Geometry check sheet. Reference: the model listing, model coordinates, mm. Give positions to 0.01 mm unless a question says otherwise; leave off trailing zeros. Write each loop counter-clockwise with the first axis right and the second up, starting at its lowest first coordinate (ties: lowest second). Pieces come first, ordered by that corner, then holes.
(1) Cross-section at D-D (y = -51). Record the boundary of the cut face in (x, z), and give its area (3 significant figures).
(2) Cross-section at A-A (x = 48). Record the boundary of the cut face in (y, z), and give its area (3 significant figures).
(3) Thickness scan on line 1 along Y through (x, z) = (48, 0.3); line 2 along Y through (x, z) = (19, 0.65); line 3 along X through (y, z) = (-25.5, 0.65). Record the ranges inside material, lowest first.
(4) Depth check by flat-ended pin: P1, Ø1.7, axis at x = 48, y = -32.46, coming from the +Z side; P2, Ø0.5, axis at y = -39, z = 0.5, coming from the -X side. Enter the tip coordinate at first touch or a pass-through.
(5) Mould release check, pull along X, two halves, no side actions. Record for faces 1 (the cylindrical face through (18.902, -29.176, 0.507)), 2 (the flat face through (34, -21, 1)): +X half, -X half, draft (parallel to the pull), parting line (faces both ways), or undercut.
(6) Cross-section at B-B (z = 0.85). Count the separate pieces of the cut face and the enclosed holes in it, and give its area (3 significant figures).
(7) Cross-section at C-C (y = -29.92). Record the boundary of the cut face in (x, z), and give its area (3 significant figures).
```python
from build123d import *

# Parameters (mm, degrees)
IZIM1_R                     = 1.6
Y_KSEKLIK_EKSTR_ZYON1_DEPTH = 1
IZIM2_R                     = 0.75
KES_EKSTR_ZYON1_DEPTH       = 10


with BuildPart() as part:
    # Çizim1 → Yükseklik-Ekstrüzyon1 (new body)
    with BuildSketch(Plane.XY):
        Polygon((0, 0), (68, 0), (68, -17), (51, -17), (51, -54), (17, -54), (17, -17), (0, -17), align=None)
        with Locations((3, -8)):
            Circle(IZIM1_R, mode=Mode.SUBTRACT)
        with Locations((66, -8)):
            Circle(IZIM1_R, mode=Mode.SUBTRACT)
        with Locations((20, -51)):
            Circle(IZIM1_R, mode=Mode.SUBTRACT)
        with Locations((48, -51)):
            Circle(IZIM1_R, mode=Mode.SUBTRACT)
    extrude(amount=Y_KSEKLIK_EKSTR_ZYON1_DEPTH)

    # Çizim2 → Kes-Ekstrüzyon1 (cut)
    with BuildSketch(Plane.XY.offset(1)):
        with Locations((19, -35)):
            Circle(IZIM2_R)
        with Locations((19, -32.46)):
            Circle(IZIM2_R)
        with Locations((19, -29.92)):
            Circle(IZIM2_R)
        with Locations((48, -29.92)):
            Circle(IZIM2_R)
        with Locations((48, -32.46)):
            Circle(IZIM2_R)
        with Locations((48, -35)):
            Circle(IZIM2_R)
    extrude(amount=-KES_EKSTR_ZYON1_DEPTH, mode=Mode.SUBTRACT)


solid = part.part
```
Reply:
1. outline: (17, 0) - (18.4, 0) - (18.4, 1) - (17, 1) - close; (21.6, 0) - (46.4, 0) - (46.4, 1) - (21.6, 1) - close; (49.6, 0) - (51, 0) - (51, 1) - (49.6, 1) - close
1. area: 27.6 mm2
2. outline: (-54, 0) - (-52.6, 0) - (-52.6, 1) - (-54, 1) - close; (-49.4, 0) - (-35.75, 0) - (-35.75, 1) - (-49.4, 1) - close; (-34.25, 0) - (-33.21, 0) - (-33.21, 1) - (-34.25, 1) - close; (-31.71, 0) - (-30.67, 0) - (-30.67, 1) - (-31.71, 1) - close; (-29.17, 0) - (0, 0) - (0, 1) - (-29.17, 1) - close
2. area: 46.3 mm2
3. line 1: y = -54 to -52.6, -49.4 to -35.75, -34.25 to -33.21, -31.71 to -30.67, -29.17 to 0
3. line 2: y = -54 to -52.25, -49.75 to -35.75, -34.25 to -33.21, -31.71 to -30.67, -29.17 to 0
3. line 3: x = 17 to 51
4. P1: stops at z = 1
4. P2: stops at x = 17
5. face 1: undercut
5. face 2: draft
6. separate pieces: 1
6. enclosed holes: 10
6. area: 2,370 mm2
7. outline: (17, 0) - (18.25, 0) - (18.25, 1) - (17, 1) - close; (19.75, 0) - (47.25, 0) - (47.25, 1) - (19.75, 1) - close; (48.75, 0) - (51, 0) - (51, 1) - (48.75, 1) - close
7. area: 31.0 mm2
